Here's how the part is built. I have some questions about the finished solid (model axes, mm). A direction names the side the tool comes from. Round coordinates to 2 decimals unless told otherwise and drop trailing zeros. Loops run counter-clockwise (first coordinate to the right, second up) from the corner with the lowest first, then second, coordinate; pieces in that order, holes last. Notation, with made-up numbers: M -12,-17 L 36,-17 A18 cw 36,3 Z; hole C -12.5,35.25 d9. An arc over 180 degrees is marked long. Put each result on its own line as item: value. Start each with the question number.
```python
from build123d import *

# Parameters (mm, degrees)
F1_DEPTH  = 20
F3_DEPTH  = 2
F0_W      = 0.4
F0_H      = 1
F4_DEPTH  = 0.8
F5_SIZE   = 0.39999
F6_R      = 5
F7_R      = 0.79999
F8_SIZE   = 1
F9_R      = 1
F10_DEPTH = 1.2


# Not quite as in the source:
# - a fillet or chamfer is up to 0.001 mm smaller than in the source, because OpenCascade refuses the exact size


with BuildPart() as f1:
    # F0 (on Front) → F1 (new body)
    with BuildSketch(Plane.XZ):
        Polygon((9.6, -5), (0, -5), (-9.6, -5), (-9.6, -2.7), (-6.35, -2.7), (-6.35, -1), (-5.2, -1), (-5.2, 0), (-11.6, 0), (-14.4, -6.2), (0, -6.2), (14.4, -6.2), (11.6, 0), (5.2, 0), (5.2, -1), (6.35, -1), (6.35, -2.7), (9.6, -2.7), align=None)
    extrude(amount=F1_DEPTH)

    # F2 (on face) → F3 (join)
    with BuildSketch(Plane.XZ.offset(20)):
        Polygon((-5.2, 0), (-11.6, 0), (-14.4, -6.2), (11.6, -6.2), (11.6, 0), (5.2, 0), (5.2, -1), (6.35, -1), (6.35, -2.7), (9.6, -2.7), (9.6, -5), (-9.6, -5), (-9.6, -2.7), (-6.35, -2.7), (-6.35, -1), (-5.2, -1), align=None)
        Polygon((5.2, 0), (-5.2, 0), (-5.2, -1), (-6.35, -1), (-6.35, -2.7), (-9.6, -2.7), (-9.6, -5), (9.6, -5), (9.6, -2.7), (6.35, -2.7), (6.35, -1), (5.2, -1), align=None)
    extrude(amount=-F3_DEPTH)

    # F0 (on Front) + F3_face (on face) + F3_face1 (on face) → F4 (join)
    with BuildSketch(Plane.XZ):
        with Locations((5, -0.5)):
            Rectangle(F0_W, F0_H)
        with Locations((-5, -0.5)):
            Rectangle(F0_W, F0_H)
    with BuildSketch(Plane(origin=(0, -18, -2.8254432042), x_dir=(1, 0, 0), z_dir=(0, 1, 0))):
        Polygon((-5.2, -2.8254432042), (5.2, -2.8254432042), (5.2, -1.8254432042), (6.35, -1.8254432042), (6.35, -0.1254432042), (9.6, -0.1254432042), (9.6, 2.1745567958), (-9.6, 2.1745567958), (-9.6, -0.1254432042), (-6.35, -0.1254432042), (-6.35, -1.8254432042), (-5.2, -1.8254432042), align=None)
    with BuildSketch(Plane(origin=(0, -20, -3.2112820513), x_dir=(1, 0, 0), z_dir=(0, -1, 0))):
        Polygon((14.4, -2.9887179487), (11.6, 3.2112820513), (-11.6, 3.2112820513), (-14.4, -2.9887179487), align=None)
    extrude(amount=F4_DEPTH, dir=(0, -1, 0))

    # F5 (size 0.4 in the source; OpenCascade refuses exactly that, so slightly less here)
    f5_edges = [f1.edges().sort_by_distance(p)[0] for p in [
        (-4.8, -0.8, -0.5),
        (4.8, -0.8, -0.5),
    ]]
    chamfer(f5_edges, length=F5_SIZE)

    # F6
    f6_edges = [f1.edges().sort_by_distance(p)[0] for p in [
        (11.6, -10.4, 0),
        (-11.6, -10.4, 0),
    ]]
    fillet(f6_edges, radius=F6_R)

    # F7 (radius 0.8 in the source; OpenCascade refuses exactly that, so slightly less here)
    f7_edges = [f1.edges().sort_by_distance(p)[0] for p in [
        (13.664338, -20.8, -4.571033),
        (13.664338, 0, -4.571033),
        (-11.083863, 0, -0.799425),
    ]]
    fillet(f7_edges, radius=F7_R)

    # F8
    f8_edges = [f1.edges().sort_by_distance(p)[0] for p in [
        (-9.6, 0, -3.85),
        (-6.35, 0, -1.85),
        (6.35, 0, -1.85),
        (9.6, 0, -3.85),
    ]]
    chamfer(f8_edges, length=F8_SIZE)

    # F9 (on face) → F10 (cut, through all)
    with BuildSketch(Plane(origin=(0, 0, -6.2), x_dir=(1, 0, 0), z_dir=(0, 0, -1))):
        with Locations((0, 10.4)):
            Circle(F9_R)
    extrude(amount=-F10_DEPTH, mode=Mode.SUBTRACT)


solid = f1.part
```
1) If we mould it in two halves opening along Z, with no side actions, what happens to faces 1 (the face through (-0.2, 0, -5.3)), 2 (the face through (-6.35, -9, -2)), 3 (the face through (-13.455, -0.228, -4.693)), 4 (the face through (0, -8, -6.2))? For each: pulls with the +Z half, pulls with the -Z half, needs draft (parallel to the pull), parting line crosses it, or undercut.
2) On a 3-axis mill with a long thin cutter (end or side, diameter ignored), from which of +Z, -Z, +X, -X, +Y, -Y can I reach the whole of each face in a straight line? I mean faces 5 (the face through (11.05, -10.27, -0.78)), 6 (the face through (-9.6, -9, -4)). Say none if no direction works.
3) Suppose I cut it at B-B (y = -10.4). Write out the boundary of the cut face in (x, z).
4) Suppose I cut it at C-C (y = -2). Write out the boundary of the cut face in (x, z), plus the area to 3 significant figures.
5) If I drill on probe 1 along Y at (x, z) = (0, -5.25); probe 2 along Z at (x, y) = (-6.5, -7); probe 3 along X at (y, z) = (-10.4, -5.9), over which ranges is the centre line in solid material (lowest first)? Write a range as from..to.
6) Suppose I cut it at D-D (x = 6). Write out the boundary of the cut face in (y, z).
7) I'm going to push flat-ended pins straight in: P1, Ø1.9, axis at y = -10, z = -2, coming from the +X side; P2, Ø1.4, axis at y = -13.5, z = -2, coming from the -X side; P3, Ø3, axis at x = -10, y = -15.5, coming from the +Z side; P4, Ø0.8, axis at y = -12.5, z = -0.5, coming from the -X side. Where does each tip first touch, or does it pass through?
8) Suppose I cut it at A-A (x = 0). Write out the boundary of the cut face in (y, z).
Results are:
1. face 1: needs draft
1. face 2: undercut
1. face 3: pulls with the +Z half
1. face 4: pulls with the -Z half
2. face 5: +Z, +X, +Y, -Y
2. face 6: +Y
3. outline: M -14.4,-6.2 L -1,-6.2 L -1,-5 L -9.6,-5 L -9.6,-2.7 L -6.35,-2.7 L -6.35,-1 L -5.2,-1 L -5.2,0 L -8.37,0 A5 ccw -12.93,-2.94 Z; M 1,-6.2 L 14.4,-6.2 L 12.93,-2.94 A5 ccw 8.37,0 L 5.2,0 L 5.2,-1 L 6.35,-1 L 6.35,-2.7 L 9.6,-2.7 L 9.6,-5 L 1,-5 Z
4. outline: M -14.4,-6.2 L 14.4,-6.2 L 12.93,-2.94 A5 ccw 8.37,0 L 5.2,0 L 5.2,-1 L 6.35,-1 L 6.35,-2.7 L 9.6,-2.7 L 9.6,-5 L -9.6,-5 L -9.6,-2.7 L -6.35,-2.7 L -6.35,-1 L -5.2,-1 L -5.2,0 L -8.37,0 A5 ccw -12.93,-2.94 Z
4. area: 81.4 mm²
5. probe 1: -20.8..-11.4, -9.4..0
5. probe 2: -6.2..-5, -2.7..0
5. probe 3: -14.26..-1, 1..14.26
6. outline: M -20.8,-6.2 L 0,-6.2 L 0,-5 L -18,-5 L -18,-1 L 0,-1 L 0,-0.8 A0.8 ccw -0.8,0 L -20,0 A0.8 ccw -20.8,-0.8 Z
7. P1: x = 12.93
7. P2: x = -12.81
7. P3: z = 0
7. P4: x = -11.23
8. outline: M -20.8,-6.2 L -11.4,-6.2 L -11.4,-5 L -18,-5 L -18,0 L -20,0 A0.8 ccw -20.8,-0.8 Z; M -9.4,-6.2 L 0,-6.2 L 0,-5 L -9.4,-5 Z
